```python
from build123d import *

# Parameters (mm, degrees)
RESSALTO_EXTRUS_O1_DEPTH      = 2
RESSALTO_EXTRUS_O3_DEPTH      = 30
RESSALTO_EXTRUS_O3_DEPTH_BACK = 2
ESBO_O2_W                     = 2
ESBO_O2_H                     = 20
ESBO_O3_R                     = 2.5
CORTE_EXTRUS_O1_DEPTH         = 2
CORTE_EXTRUS_O2_DEPTH         = 50.244289009
CORTE_EXTRUS_O2_DEPTH_BACK    = 50.244289009
ESBO_O4_R                     = 2.5


with BuildPart() as part:
    # Esboço1 → Ressalto-extrusão1 (new body)
    with BuildSketch(Plane(origin=(0, 0, 0), x_dir=(1, 0, 0), z_dir=(0, 1, 0))):
        Polygon((10, 10), (10, -10), (25, -10), (25, -30), (-25, -30), (-25, -10), (-10, -10), (-10, 10), (-25, 10), (-25, 30), (25, 30), (25, 10), align=None)
    extrude(amount=-RESSALTO_EXTRUS_O1_DEPTH)

    # Esboço2 → Ressalto-extrusão3 (add, two sides: drawn at the far end of the back side and taken through both)
    with BuildSketch(Plane(origin=(0, 0, 0), x_dir=(1, 0, 0), z_dir=(0, 1, 0)).offset(-RESSALTO_EXTRUS_O3_DEPTH_BACK)):
        with Locations((-11, 0)):
            Rectangle(ESBO_O2_W, ESBO_O2_H)
        with Locations((11, 0)):
            Rectangle(ESBO_O2_W, ESBO_O2_H)
    extrude(amount=RESSALTO_EXTRUS_O3_DEPTH + RESSALTO_EXTRUS_O3_DEPTH_BACK)

    # Esboço3 → Corte-extrusão1 (cut)
    with BuildSketch(Plane(origin=(0, 0, 0), x_dir=(1, 0, 0), z_dir=(0, 1, 0))):
        with Locations(Location((16, -22, 0), (0, 0, 270))):
            Circle(ESBO_O3_R)
        with Locations(Location((-16, -22, 0), (0, 0, 270))):
            Circle(ESBO_O3_R)
        with Locations(Location((5, -5, 0), (0, 0, 270))):
            Circle(ESBO_O3_R)
        with Locations(Location((-5, 5, 0), (0, 0, 270))):
            Circle(ESBO_O3_R)
        with Locations(Location((16, 22, 0), (0, 0, 270))):
            Circle(ESBO_O3_R)
        with Locations(Location((-16, 22, 0), (0, 0, 270))):
            Circle(ESBO_O3_R)
    extrude(amount=-CORTE_EXTRUS_O1_DEPTH, mode=Mode.SUBTRACT)

    # Esboço4 → Corte-extrusão2 (cut, two sides: drawn at the far end of the back side and taken through both)
    with BuildSketch(Plane(origin=(0, 0, 0), x_dir=(0, 0, -1), z_dir=(1, 0, 0)).offset(-CORTE_EXTRUS_O2_DEPTH_BACK)):
        with Locations((0, 25)):
            Circle(ESBO_O4_R)
    extrude(amount=CORTE_EXTRUS_O2_DEPTH + CORTE_EXTRUS_O2_DEPTH_BACK, mode=Mode.SUBTRACT)


solid = part.part
```
For this review, take the finished solid that the model builds, in its own axes (mm). A direction names the side the tool comes from. Coordinates: 2 decimals unless noted, no trailing zeros. Loops run counter-clockwise (first coordinate to the right, second up) from the corner with the lowest first, then second, coordinate; pieces in that order, holes last. Notation, with made-up numbers: (-1, 89) -> (55, 89) arc R31 ccw to (55, 128) -> close; hole circle Ø1 at (77.25, -8.75). An arc over 180 degrees is marked (long way). Return JSON: item names as keys, results as strings. Group by question number.
(1) To check wall thickness, follow L1, parallel to X at y = -1, z = 22; L2, parallel to Z at x = -11.05, y = 25; L3, parallel to Y at x = -11.2, z = 0. State the ranges of each line that lie inside material, in increasing order.
(2) Consider section C-C, the plane x = -5. Give the boundary of the cut face in (y, z).
(3) Consider section A-A, the plane z = 22. Give the boundary of the cut face in (x, y), plus the area to 3 significant figures.
(4) Consider section D-D, the plane z = 5. Give the boundary of the cut face in (x, y).
(5) For pin 1 Ø1.5 at (y, z) = (19.5, 10) entering from +X; pin 2 Ø1.6 at (x, y) = (10.5, 14.5) entering from -Z; pin 3 Ø10 at (x, y) = (11.5, 24.5) entering from +Z; pin 4 Ø6 at (x, y) = (2.5, 3.5) entering from +Z, all flat-tipped, find the tip position at first contact; note any pin that passes through.
(6) Consider section B-B, the plane y = 26.5. Give the boundary of the cut face in (x, z), plus the area to 3 significant figures.
(7) Mouldability with a two-part tool opening along Y and no side actions: class faces 5 (the cylindrical face through (10.99, 27.48, 0.33)), 6 (the flat face through (-11, 30, 0)), 7 (the flat face through (0, -1, 30)), 8 (the flat face through (0, -2, 0)) as pulls with the +Y half, pulls with the -Y half, needs draft (parallel to the pull), parting line crosses it, or undercut.
(8) Tool access review of faces 1 (the flat face through (25, -1, 20)), 2 (the flat face through (11, 15, -10)), 3 (the flat face through (-10, 15, 0)), 4 (the flat face through (-11, 15, 10)): name each direction out of +Z, -Z, +X, -X, +Y, -Y from which nothing blocks a thin tool from reaching the whole face with its end or side.
Results below:
{
 "1": {"L1": "x = -25 to -18.5, -13.5 to 13.5, 18.5 to 25", "L2": "z = -10 to -2.5, 2.5 to 10", "L3": "y = -2 to 22.5, 27.5 to 30"},
 "2": {"outline": "(-2, -30) -> (0, -30) -> (0, -7.5) -> (-2, -7.5) -> close; (-2, -2.5) -> (0, -2.5) -> (0, 30) -> (-2, 30) -> close"},
 "3": {"outline": "(-25, -2) -> (-18.5, -2) -> (-18.5, 0) -> (-25, 0) -> close; (-13.5, -2) -> (13.5, -2) -> (13.5, 0) -> (-13.5, 0) -> close; (18.5, -2) -> (25, -2) -> (25, 0) -> (18.5, 0) -> close", "area": "80.0 mm2"},
 "4": {"outline": "(-12, -2) -> (2.5, -2) -> (2.5, 0) -> (-10, 0) -> (-10, 30) -> (-12, 30) -> close; (7.5, -2) -> (12, -2) -> (12, 30) -> (10, 30) -> (10, 0) -> (7.5, 0) -> close"},
 "5": {"pin 1": "stops at x = 12", "pin 2": "stops at z = -10", "pin 3": "stops at z = 10", "pin 4": "passes through"},
 "6": {"outline": "(-12, -10) -> (-10, -10) -> (-10, -2) -> (-12, -2) -> close; (-12, 2) -> (-10, 2) -> (-10, 10) -> (-12, 10) -> close; (10, -10) -> (12, -10) -> (12, -2) -> (10, -2) -> close; (10, 2) -> (12, 2) -> (12, 10) -> (10, 10) -> close", "area": "64.0 mm2"},
 "7": {"face 5": "undercut", "face 6": "pulls with the +Y half", "face 7": "needs draft", "face 8": "pulls with the -Y half"},
 "8": {"face 1": "+Z, -Z, +X, +Y, -Y", "face 2": "-Z, +X, -X, +Y", "face 3": "+Z, -Z, +Y", "face 4": "+Z, +X, -X, +Y"}
}
